```python
from build123d import *

# Parameters (mm, degrees)
SKETCH1_W                                = 10
SKETCH1_H                                = 31
BOSS_EXTRUDE1_DEPTH                      = 10
SKETCH2_W                                = 3
SKETCH2_H                                = 5.5
CUT_EXTRUDE1_DEPTH                       = 10
CBORE_FOR_M2_PAN_HEAD_SCREW1_D           = 2.4
CBORE_FOR_M2_PAN_HEAD_SCREW1_DEPTH       = 10
CBORE_FOR_M2_PAN_HEAD_SCREW1_CBORE_D     = 5
CBORE_FOR_M2_PAN_HEAD_SCREW1_CBORE_DEPTH = 1.6
CBORE_FOR_M2_PAN_HEAD_SCREW1_TIP         = 0.721032743


with BuildPart() as part:
    # Sketch1 → Boss-Extrude1 (new body)
    with BuildSketch(Plane.XY):
        with Locations((5, 15.5)):
            Rectangle(SKETCH1_W, SKETCH1_H)
    extrude(amount=BOSS_EXTRUDE1_DEPTH)

    # Sketch2 → Cut-Extrude1 (cut)
    with BuildSketch(Plane.XY.offset(10)):
        with Locations((1.5, 28.25)):
            Rectangle(SKETCH2_W, SKETCH2_H)
    extrude(amount=-CUT_EXTRUDE1_DEPTH, mode=Mode.SUBTRACT)

    # CBORE for M2 Pan Head Screw1
    with Locations(Plane.XY.offset(10)):
        with Locations((5, 14), (5, 6)):
            CounterBoreHole(CBORE_FOR_M2_PAN_HEAD_SCREW1_D / 2, CBORE_FOR_M2_PAN_HEAD_SCREW1_CBORE_D / 2, CBORE_FOR_M2_PAN_HEAD_SCREW1_CBORE_DEPTH, depth=CBORE_FOR_M2_PAN_HEAD_SCREW1_DEPTH)
            with Locations((0, 0, -(CBORE_FOR_M2_PAN_HEAD_SCREW1_DEPTH + CBORE_FOR_M2_PAN_HEAD_SCREW1_TIP / 2))):  # 118° drill point
                Cone(0, CBORE_FOR_M2_PAN_HEAD_SCREW1_D / 2, CBORE_FOR_M2_PAN_HEAD_SCREW1_TIP, mode=Mode.SUBTRACT)


solid = part.part
```
Part model, mm, in its own coordinate system. A direction names the side the tool comes from. Give positions to 0.01 mm unless a question says otherwise; leave off trailing zeros. Order: outer loops, then holes, each group sorted by start corner. A loop starts at its lowest first (then second) coordinate and runs counter-clockwise, first axis right, second up. Notation, with made-up numbers: M 72.25,37 L 90.25,37 A23 cw 90.25,63 Z; hole C -15.5,43.5 d10. An arc over 180 degrees is marked long. Use a Markdown table: item, result. Add a question column.
(1) Probe line 1 along Y through (x, z) = (5, 9.35); line 2 along Y through (x, z) = (5, 2); line 3 along X through (y, z) = (14, 3.5). List the from-to ranges inside material, lowest first. Write a range as [from, to].
(2) Drop flat-ended pins along their axis: P1, Ø4, axis at x = 5, y = 14, coming from the +Z side; P2, Ø3, axis at y = 28.5, z = 4.5, coming from the -X side; P3, Ø0.9, axis at x = 1, z = 2.5, coming from the +Y side; P4, Ø1.9, axis at x = 5, y = 6, coming from the +Z side. Give the stop position or say it passes through.
(3) Saw through at D-D, the plane x = 3.5. Give the cut face in (y, z).
(4) Saw through at B-B, the plane x = 5. Give the cut face in (y, z), and give its area (3 significant figures).
(5) Saw through at A-A, the plane y = 6. Give the cut face in (x, z).
(6) Saw through at C-C, the plane z = 9.25. Give the cut face in (x, y).
(7) Mould opens along X. For faces 4 (the face through (6.15, 11.78, 9.21)), 5 (the face through (6, 31, 5)), 6 (the face through (10, 15, 5)) say: +X half, -X half, draft (parallel to the pull), parting line (faces both ways), or undercut.
(8) 3-axis set-ups, long thin cutter, end or side, ignore diameter. For faces 1 (the face through (6.2, 6.05, 4.14)), 2 (the face through (7.385, 6.751, 9.211)), 3 (the face through (3, 28, 5)): which of +Z, -Z, +X, -X, +Y, -Y reach the whole face in a straight line?
Answer key:
| question | item | result |
|---|---|---|
| 1 | line 1 | [0, 3.5], [8.5, 11.5], [16.5, 31] |
| 1 | line 2 | [0, 4.8], [7.2, 12.8], [15.2, 31] |
| 1 | line 3 | [0, 3.8], [6.2, 10] |
| 2 | P1 | z = 8.4 |
| 2 | P2 | x = 3 |
| 2 | P3 | y = 25.5 |
| 2 | P4 | through |
| 3 | outline | M 0,0 L 31,0 L 31,10 L 16,10 L 16,8.4 L 12,8.4 L 12,10 L 8,10 L 8,8.4 L 4,8.4 L 4,10 L 0,10 Z |
| 4 | outline | M 0,0 L 4.8,0 L 4.8,8.4 L 3.5,8.4 L 3.5,10 L 0,10 Z; M 7.2,0 L 12.8,0 L 12.8,8.4 L 11.5,8.4 L 11.5,10 L 8.5,10 L 8.5,8.4 L 7.2,8.4 Z; M 15.2,0 L 31,0 L 31,10 L 16.5,10 L 16.5,8.4 L 15.2,8.4 Z |
| 4 | area | 254 mm^2 |
| 5 | outline | M 0,0 L 3.8,0 L 3.8,8.4 L 2.5,8.4 L 2.5,10 L 0,10 Z; M 6.2,0 L 10,0 L 10,10 L 7.5,10 L 7.5,8.4 L 6.2,8.4 Z |
| 6 | outline | M 0,0 L 10,0 L 10,31 L 3,31 L 3,25.5 L 0,25.5 Z; hole C 5,6 d5; hole C 5,14 d5 |
| 7 | face 4 | undercut |
| 7 | face 5 | draft |
| 7 | face 6 | +X half |
| 8 | face 1 | +Z, -Z |
| 8 | face 2 | +Z |
| 8 | face 3 | +Z, -Z, -X, +Y |
